Autodesk Fusion 360 part; units mm, degrees
sketch "Sketch1" plane through (0, 0, 0) normal (0, 1, 0) x (1, 0, 0)
  line L0 (0, 0) -> (0, -20)
  line L1 (0, 0) -> (155, 0)
  line L2 (155, 0) -> (155, 20)
  line L3 (155, 20) -> (182.5, 20)
  line L4 (182.5, 20) -> (182.5, 36)
  line L5 (182.5, 36) -> (204.5, 36)
  line L6 (204.5, 36) -> (204.5, 41)
  line L7 (204.5, 41) -> (104.5, 41)
  dimension "d1" = 20
  dimension "d2" = 155
  dimension "d11" = 20
  dimension "d12" = 27.5
  dimension "d13" = 16
  dimension "d14" = 22
  dimension "d15" = 5
  dimension "d16" = 100
sketch "Sketch2" plane through (0, 0, 0) normal (1, 0, 0) x (0, 1, 0)
  line L0 (0, 0) -> (0, 20)
  line L1 (0, 20) -> (0, 37.25) construction
  circle A0 centre (0, 37.25) radius 17.25
  circle A1 centre (0, 37.25) radius 15.75
  point P0 (0, 20)
  dimension "d3" = 17.25
  dimension "d4" = -1.5
ref_plane "WorkPlane1" through (20, 0, 0) normal (1, 0, 0) x (0, 1, 0)
sketch "Sketch3" plane through (20, 0, 0) normal (1, 0, 0) x (0, 1, 0)
  circle A0 centre (0, 37.25) radius 15.75 construction
  circle A1 centre (0, 37.25) radius 17.9
  circle A2 centre (0, 37.25) radius 16.4
  dimension "d6" = 35.8
  dimension "d7" = -1.5
loft "Loft1" add profiles "Sketch2", "Sketch3" section 1 section 2
loft "Loft2" cut profiles "Sketch3", "Sketch2" section 1 contours A2 section 2 contours A1
ref_plane "WorkPlane2" through (35, 0, 37.25) normal (1, 0, 0) x (0, 1, 0)
sketch "Sketch4" plane through (35, 0, 0) normal (1, 0, 0) x (0, 1, 0)
  circle A0 centre (0, 37.25) radius 16.4 construction
  circle A1 centre (0, 37.25) radius 29.25
  circle A2 centre (0, 37.25) radius 31.25
  dimension "d9" = 58.5
  dimension "d10" = 2
loft "Loft3" add profiles "Sketch3", "Sketch4" section 1 contours A1 | A2 section 2 contours A1 | A2
loft "Loft4" cut profiles "Sketch4", "Sketch3" section 1 contours A1 section 2 contours A2
extrude "Extrude1" add sketch "Sketch4" along normal blind 120
fillet "Fillet1" radius 10 2 edges at (20, -15.2902, 43.1805) (20, -16.6887, 43.7229)
fillet "Fillet2" radius 15 2 edges at (35, -27.2706, 47.8273) (35, -29.1352, 48.5505)
equation "d3 = ( 34.5 / 2 ) * 1 mm"
Check sheet for the modelled part. Datum: model origin and axes. Units: mm. Round coordinates to 2 decimals unless told otherwise and drop trailing zeros. Loops run counter-clockwise (first coordinate to the right, second up) from the corner with the lowest first, then second, coordinate; pieces in that order, holes last. Notation, with made-up numbers: M 25,-16.75 L 42,-16.75 A21 cw 42,22.25 Z; hole C -40,40.5 d6. An arc over 180 degrees is marked long. One line per item, written item: value.
(1) Sectioned sample at A-A, the plane x = 76. Record the cut outline in (y, z), then the cut area to 3 significant figures.
Computed values:
outline: C 0,37.25 d62.5; hole C 0,37.25 d58.5
area: 380 mm^2
(2) Depth check by flat-ended pin: pin 1 Ø1.5 at (y, z) = (-17, 57.5) entering from +X; pin 2 Ø5 at (y, z) = (-1, 26) entering from -X; pin 3 Ø5 at (x, z) = (110.5, 24) entering from +Y; pin 4 Ø1.5 at (x, y) = (28.5, 15) entering from -Z. Enter the tip coordinate at first touch or a pass-through.
Computed values:
pin 1: stops at x = 32.96
pin 2: passes through
pin 3: stops at y = 29.34
pin 4: stops at z = 15.7
(3) Thickness scan on line 1 (Y direction, x = 75.5, z = 37.25); line 2 (Z direction, x = 73, y = 0); line 3 (Y direction, x = 109.5, z = 27). Record the ranges inside material, lowest first.
Computed values:
line 1: y = -31.25 to -29.25, 29.25 to 31.25
line 2: z = 6 to 8, 66.5 to 68.5
line 3: y = -29.52 to -27.4, 27.4 to 29.52
(4) Release check for a two-part mould opening along Z. For faces 1 (the face through (0, 14, 29.7)), 2 (the face through (23.21, -2.7, 57.83)), 3 (the face through (96.972, -6.341, 65.804)) record: +Z half, -Z half, draft (parallel to the pull), parting line (faces both ways), or undercut.
Computed values:
face 1: draft
face 2: parting line
face 3: undercut
